Here's how the part is built. I have some questions about the finished solid (model axes, mm). A direction names the side the tool comes from. Round coordinates to 2 decimals unless told otherwise and drop trailing zeros. Order: outer loops, then holes, each group sorted by start corner. A loop starts at its lowest first (then second) coordinate and runs counter-clockwise, first axis right, second up. Notation, with made-up numbers: M 44.5,23.5 L 92.5,23.5 A22 cw 92.5,50.5 Z; hole C 35.5,75 d1. An arc over 180 degrees is marked long. Write item = value, one per line. Start each with the question number.
Item 1: I want a section at B-B, the plane z = 1.25. List the corners of the cut face in (x, y) for me.
Item 2: I'm going to push flat-ended pins straight in: P1, Ø4, axis at y = 11, z = 5.5, coming from the -X side; P2, Ø2, axis at y = 3, z = 4.5, coming from the -X side; P3, Ø5, axis at x = -16.5, z = 3.5, coming from the -Y side. Where does each tip first touch, or does it pass through?
Item 3: We'd pull the mould along Y, two halves only. Please class faces 6 (the face through (-9, 14, 5)), 7 (the face through (-52.73, 80.35, 4.93)), 8 (the face through (-3, 0, 5)): pulls with the +Y half, pulls with the -Y half, needs draft (parallel to the pull), parting line crosses it, or undercut.
Item 4: I want a section at A-A, the plane y = 14. List the corners of the cut face in (x, z) for me.
Item 5: Please list where these lines run through material, in increasing order: L1, parallel to X at y = 23.5, z = 8; L2, parallel to Y at x = -5.5, z = 6.75; L3, parallel to X at y = 18, z = 1.5.
Item 6: I want a section at C-C, the plane x = -38. List the corners of the cut face in (y, z) for me.
Item 7: I want a section at D-D, the plane y = 54.5. List the corners of the cut face in (x, z) for me, plus the area to 3 significant figures.
Item 8: For faces 1 (the face through (-19, 41, 0)), 2 (the face through (-25, 23, 5)), 3 (the face through (-7.5, 6, 5)), 4 (the face through (-6, 12.5, 5)), 5 (the face through (-15, 20, 5)), which set-ups out of +Z, -Z, +X, -X, +Y, -Y let a thin tool reach every point of the face, with its end or its side?
```python
from build123d import *

# Parameters (mm, degrees)
F1_DEPTH = 10
F2_R     = 5
F3_R     = 1.65
F4_DEPTH = 58.3841123594
F5_DEPTH = 25


with BuildPart() as f1:
    # F0 (on Top) → F1 (new body)
    with BuildSketch(Plane.XY):
        Polygon((-25, 25), (-25, 20), (-5, 20), (-5, 12.5), (-7.5, 12.5), (-7.5, 15), (-8, 15), (-10.5, 12.5), (-10.5, 7.5), (-8, 5), (-7.5, 5), (-7.5, 7.5), (-5, 7.5), (-5, 0), (0, 0), (0, 26.9574919131), (-50.9201724728, 82.0223267475), (-54.5911614618, 78.6276485826), (-5, 25), align=None)
    extrude(amount=F1_DEPTH)

    # F2
    f2_edges = [f1.edges().sort_by_distance(p)[0] for p in [
        (-5, 25, 5),
    ]]
    fillet(f2_edges, radius=F2_R)

    # F3 (on face) → F4 (cut, through all)
    with BuildSketch(Plane(origin=(13.4375831218, 12.4261527749, 0), x_dir=(-0.678935633, 0.7341977978, 0), z_dir=(0.7341977978, 0.678935633, 0))):
        with Locations((89.7921311966, 5)):
            Circle(F3_R)
    extrude(amount=-F4_DEPTH, mode=Mode.SUBTRACT)

    # F3 (on face) → F5 (cut)
    with BuildSketch(Plane(origin=(13.4375831218, 12.4261527749, 0), x_dir=(-0.678935633, 0.7341977978, 0), z_dir=(0.7341977978, 0.678935633, 0))):
        with Locations((39.7921311966, 5)):
            Circle(F3_R)
    extrude(amount=-F5_DEPTH, mode=Mode.SUBTRACT)


solid = f1.part
```
Filled in:
q1.outline = M -54.59,78.63 L -12.76,33.39 A5 cw -16.43,25 L -25,25 L -25,20 L -5,20 L -5,12.5 L -7.5,12.5 L -7.5,15 L -8,15 L -10.5,12.5 L -10.5,7.5 L -8,5 L -7.5,5 L -7.5,7.5 L -5,7.5 L -5,0 L 0,0 L 0,26.96 L -50.92,82.02 Z
q2.P1 = -10.5
q2.P2 = -5
q2.P3 = 20
q3.face_6 = undercut
q3.face_7 = pulls with the +Y half
q3.face_8 = pulls with the -Y half
q4.outline = M -9,0 L -7.5,0 L -7.5,10 L -9,10 Z; M -5,0 L 0,0 L 0,10 L -5,10 Z
q5.L1 = -25 to 0
q5.L2 = 7.5 to 12.5, 20 to 32.91
q5.L3 = -5 to 0
q6.outline = M 60.69,0 L 68.05,0 L 68.05,10 L 60.69,10 Z
q7.outline = M -32.28,0 L -25.47,0 L -25.47,10 L -32.28,10 Z
q7.area = 68.1 mm^2
q8.face_1 = -Z, +X, -X, +Y, -Y
q8.face_2 = +Z, -Z, -X, -Y
q8.face_3 = +Z, -Z, -Y
q8.face_4 = +Z, -Z
q8.face_5 = +Z, -Z, -X
